Verification items for the finished model (mm, model axes). A direction names the side the tool comes from. Coordinates: 2 decimals unless noted, no trailing zeros. Write each loop counter-clockwise with the first axis right and the second up, starting at its lowest first coordinate (ties: lowest second). Pieces come first, ordered by that corner, then holes. Notation, with made-up numbers: M 27,33 L 65,33 A24 ccw 65,70 Z; hole C 14.5,77.25 d3. An arc over 180 degrees is marked long. One line per item, written item: value.
Autodesk Inventor part; units mm, degrees
ref_plane "YZ Plane" through (0, 0, 0) normal (1, 0, 0) x (0, 1, 0)
ref_plane "XZ Plane" through (0, 0, 0) normal (0, 1, 0) x (-1, 0, 0)
ref_plane "XY Plane" through (0, 0, 0) normal (0, 0, 1) x (1, 0, 0)
sketch "Sketch1" plane through (0, 0, 0) normal (0, 1, 0) x (-1, 0, 0)
  line L0 (0, 0) -> (-94, 0)
  line L1 (-94, 0) -> (-94, -87)
  line L2 (-94, -87) -> (0, -87)
  line L3 (0, -87) -> (0, 0)
  dimension "d0" = 94
  dimension "d1" = 87
extrude "Extrusion1" add sketch "Sketch1" along normal blind 2
sketch "Sketch2" plane through (0, 0, 0) normal (0, 0, 1) x (1, 0, 0)
  line L0 (94, 2) -> (0, 2)
  line L1 (-0.0001, 2) -> (94, 2)
  line L2 (94, 2) -> (99, 7)
  line L3 (94, 2) -> (101.071, 2) construction
  line L4 (94, 0) -> (99, 5)
  line L5 (99, 5) -> (114, 5)
  line L6 (114, 5) -> (114, 7)
  line L7 (114, 7) -> (99, 7)
  line L8 (94, 0) -> (94, 2)
  line L9 (94, 0) -> (94, 2)
  point P0 (0, 0)
  dimension "d4" = 7.071
  dimension "d5" = 45
  dimension "d6" = 7.071
  dimension "d7" = 15
  dimension "d8" = 2
extrude "Extrusion2" add sketch "Sketch2" against normal blind 87
sketch "Sketch3" plane through (99, 7, 0) normal (0, 1, 0) x (1, 0, 0)
  line L0 (15, 0) -> (0, 0)
  line L1 (15, 0) -> (20, 5)
  line L2 (15, 0) -> (22.071, 0) construction
  line L3 (20, 5) -> (20, 82)
  line L4 (0, 87) -> (15, 87)
  line L5 (20, 82) -> (15, 87)
  line L6 (15, 0) -> (15, 87)
  point P0 (-99, 0)
  dimension "d11" = 7.071
  dimension "d12" = 45
  dimension "d13" = 77
extrude "Extrusion3" add sketch "Sketch3" against normal blind 2
sketch "Sketch4" plane through (0, 2, 0) normal (0, 1, 0) x (1, 0, 0)
  line L0 (0, 0) -> (94, 0)
  line L1 (0, 0) -> (0, 4)
  line L2 (0, 87) -> (0, 0)
  line L3 (0, 4) -> (94, 4)
  line L4 (0, 4) -> (44, 4)
  line L5 (44, 4) -> (44, 14)
  line L6 (44, 14) -> (69, 14)
  line L7 (69, 14) -> (69, 4)
  dimension "d16" = 4
  dimension "d17" = 44
  dimension "d18" = 10
  dimension "d19" = 25
extrude "Extrusion4" cut sketch "Sketch4" against normal blind 10
ref_plane "Work Plane1" through (0, -2, 0) normal (0, -1, 0) x (1, 0, 0)
sketch "Sketch6" plane through (0, -2, 0) normal (0, -1, 0) x (1, 0, 0)
  line L0 (44, -4) -> (44, -14)
  line L1 (44, -4) -> (44, -2)
  line L2 (0, 0) -> (94, 0)
  line L3 (44, -2) -> (42, -2)
  line L4 (42, -2) -> (71, -2)
  line L5 (71, -2) -> (71, -16)
  line L6 (71, -16) -> (42, -16)
  line L7 (42, -16) -> (42, -2)
  line L8 (44, -4) -> (69, -4)
  line L9 (44, -14) -> (69, -14)
  line L10 (69, -14) -> (69, -4)
  line L11 (69, -4) -> (44, -4)
  line L12 (44, -4) -> (44, -14)
  dimension "d23" = 2
  dimension "d24" = 2
  dimension "d25" = 29
  dimension "d26" = 14
extrude "Extrusion5" add sketch "Sketch6" against normal blind 2
chamfer "Chamfer1" distance 2 angle 45 4 edges at (44, 2, -9) (56.5, 2, -14) (69, 2, -9) (56.5, 2, -4)
sketch "Sketch8" plane through (0, 2, 0) normal (0, 1, 0) x (1, 0, 0)
  line L0 (0, 0) -> (0, 25)
  line L1 (0, 87) -> (0, 0)
  line L2 (0, 25) -> (30, 25)
  circle A0 centre (30, 25) radius 7.5
  line L3 (30, 17.5) -> (30, 32.5)
  line L4 (37.5, 25) -> (22.5, 25)
  circle A1 centre (30, 25) radius 6
  line L5 (37.5, 25) -> (30, 25)
  line L6 (30, 25) -> (24, 25)
  line L7 (30, 25) -> (33.75, 25)
  line L8 (30, 25) -> (31.875, 25)
  line L9 (30, 25) -> (30.9375, 25)
  line L10 (30.9375, 25) -> (30.9375, 32.4412)
  line L11 (30.9375, 25) -> (28.9715, 25)
  line L12 (28.9715, 25) -> (28.9715, 32.4291)
  line L13 (30.9375, 25) -> (30.9375, 17.5588)
  line L14 (28.9715, 25) -> (28.9715, 17.5709)
  line L15 (30, 25) -> (30, 24.017)
  line L16 (30, 24.017) -> (30, 25.983)
  line L17 (37.4353, 25.983) -> (22.5647, 25.983)
  line L18 (37.4353, 24.017) -> (22.5647, 24.017)
  point P0 (30.9375, 24.017)
  point P1 (30.9375, 25.983)
  point P2 (28.9715, 25.983)
  point P3 (28.9715, 24.017)
  point P4 (24.0811, 25.983)
  point P5 (28.9715, 30.9112)
  point P6 (24.0811, 24.017)
  point P7 (28.9715, 19.0888)
  point P8 (35.9189, 24.017)
  point P9 (30.9375, 19.0737)
  point P10 (35.9189, 25.983)
  point P11 (30.9375, 30.9263)
  dimension "d34" = 15
  dimension "d35" = 12
  dimension "d32" = 25
  dimension "d33" = 30
  dimension "d36" = 1.966
  dimension "d37" = 0.983
  dimension "d38" = 1.966
extrude "Extrusion6" cut sketch "Sketch8" against normal blind 2 contours A0 L12 A1 L17 | L18 A1 L14 A0 | L12 L17 L3 L2 | L2 L3 L18 L14 | L4 L13 L18 L3 | L3 L17 L10 L4 | A0 L17 A1 L10 | L13 A1 L18 A0
sketch "Sketch9" plane through (0, 2, 0) normal (0, 1, 0) x (1, 0, 0)
  line L0 (0, 0) -> (0, 43)
  line L1 (0, 87) -> (0, 0)
  line L2 (0, 43) -> (21, 43)
  circle A0 centre (21, 43) radius 2.5
  line L3 (0, 0) -> (0, 52)
  line L4 (0, 52) -> (21, 52)
  circle A1 centre (21, 52) radius 2.5
  line L5 (0, 0) -> (0, 65)
  line L6 (0, 65) -> (21, 65)
  circle A2 centre (21, 65) radius 5
  dimension "d41" = 43
  dimension "d42" = 21
  dimension "d43" = 90
  dimension "d44" = 5
  dimension "d45" = 52
  dimension "d46" = 5
  dimension "d47" = 65
  dimension "d48" = 21
  dimension "d49" = 10
extrude "Extrusion7" cut sketch "Sketch9" against normal blind 2
sketch "Sketch10" plane through (0, 2, 0) normal (0, 1, 0) x (1, 0, 0)
  line L0 (0, 87) -> (0, 0)
  line L1 (0, 0) -> (43, 0)
  line L2 (0, 0) -> (94, 0)
  line L3 (43, 0) -> (43, 45)
  line L4 (71, 2) -> (42, 2)
  line L5 (71, 2) -> (70, 2)
  line L6 (70, 2) -> (70, 45)
  line L7 (70, 45) -> (74, 45) construction
  line L8 (70, 45) -> (70, 65)
  line L9 (70, 45) -> (90, 45) construction
  line L10 (70, 65) -> (67.7057, 68.2766)
  line L11 (67.7057, 68.2766) -> (45.2943, 68.2766)
  line L12 (43, 45) -> (43, 65)
  line L13 (43, 65) -> (45.2943, 68.2766)
  line L14 (70, 45) -> (70, 25)
  line L15 (70, 25) -> (66.8775, 22.5)
  line L16 (43, 45) -> (43, 25)
  line L17 (43, 25) -> (46.1225, 22.5)
  line L18 (46.1225, 22.5) -> (66.8775, 22.5)
  line L19 (66.8775, 22.5) -> (66.8775, 24.5)
  line L20 (70, 25) -> (68, 25)
  line L21 (68, 25) -> (66.8775, 24.5)
  line L22 (70, 65) -> (68, 65)
  line L23 (67.7057, 68.2766) -> (67.7057, 66.2766)
  line L24 (45.2943, 68.2766) -> (45.2943, 66.2766)
  line L25 (43, 65) -> (45, 65)
  line L26 (46.1225, 22.5) -> (46.1225, 24.5)
  line L27 (43, 25) -> (45, 25)
  line L28 (45, 25) -> (45, 65)
  line L29 (45, 65) -> (45.2943, 66.2766)
  line L30 (45.2943, 66.2766) -> (67.7057, 66.2766)
  line L31 (67.7057, 66.2766) -> (68, 65)
  line L32 (68, 65) -> (68, 25)
  line L33 (66.8775, 24.5) -> (46.1225, 24.5)
  line L34 (46.1225, 24.5) -> (45, 25)
  dimension "d52" = 43
  dimension "d53" = 45
  dimension "d54" = 1
  dimension "d58" = 20
  dimension "d59" = 90
  dimension "d60" = 20
  dimension "d61" = 4
  dimension "d62" = 20
  dimension "d63" = 4
  dimension "d64" = 2
  dimension "d65" = 2
  dimension "d66" = 2
  dimension "d67" = 2
  dimension "d68" = 2
  dimension "d69" = 2
  dimension "d70" = 2
  dimension "d71" = 2
extrude "Extrusion8" cut sketch "Sketch10" against normal blind 2 contours L28 L29 L30 L31 L32 L21 L33 L34
chamfer "Chamfer2" distance 2 angle 45 8 edges at (45, 2, -45) (45.5612, 2, -24.75) (56.5, 2, -24.5) (67.4388, 2, -24.75) (68, 2, -45) (56.5, 2, -66.2766) (45.1472, 2, -65.6383) (67.8528, 2, -65.6383)
sketch "Sketch11" plane through (0, 2, 0) normal (0, 1, 0) x (1, 0, 0)
  line L0 (45.6972, 22.5) -> (67.3028, 22.5)
  line L1 (67.3028, 22.5) -> (45.6972, 22.5)
  line L2 (43, 23.7014) -> (45.6972, 22.5)
  line L3 (45.6972, 22.5) -> (43, 23.7014)
  line L4 (43, 23.7014) -> (45, 25)
  line L5 (43, 65.2276) -> (43, 23.7014)
  line L6 (43, 23.7014) -> (43, 65.2276)
  line L7 (43.7029, 68.2766) -> (45.2943, 66.2766)
  line L8 (43, 65.2276) -> (43.7029, 68.2766)
  line L9 (70, 23.7014) -> (70, 65.2276)
  line L10 (43, 23.7014) -> (70, 23.7014)
  line L11 (70, 65.2276) -> (68, 65)
  line L12 (43, 65.2276) -> (70, 65.2276)
  line L13 (69.2971, 68.2766) -> (43.7029, 68.2766)
  line L14 (43.7029, 68.2766) -> (69.2971, 68.2766)
  line L15 (45.6972, 22.5) -> (67.3028, 22.5)
  line L16 (43, 65.2276) -> (43.7029, 68.2766)
  line L17 (43.7029, 68.2766) -> (69.2971, 68.2766)
  line L18 (46.1225, 24.5) -> (66.8775, 24.5)
  line L19 (66.8775, 24.5) -> (46.1225, 24.5)
  line L20 (45.6972, 22.5) -> (43, 23.7014)
  line L21 (43, 23.7014) -> (43, 65.2276)
  line L22 (43, 65.2276) -> (43.7029, 68.2766)
  line L23 (69.2971, 68.2766) -> (43.7029, 68.2766)
  line L24 (70, 65.2276) -> (69.2971, 68.2766)
  line L25 (69.2971, 68.2766) -> (70, 65.2276)
  line L26 (67.3028, 22.5) -> (70, 23.7014)
  line L27 (67.3028, 22.5) -> (70, 23.7014)
  line L28 (68, 25) -> (68, 65)
  line L29 (66.8775, 24.5) -> (68, 25)
  line L30 (68, 65) -> (68, 25)
  line L31 (66.8775, 24.5) -> (46.1225, 24.5)
  line L32 (45, 25) -> (46.1225, 24.5)
  line L33 (46.1225, 24.5) -> (45, 25)
  line L34 (45, 25) -> (45, 65)
  line L35 (45, 65) -> (45.2943, 66.2766)
  line L36 (67.7057, 66.2766) -> (45.2943, 66.2766)
  line L37 (68, 65) -> (67.7057, 66.2766)
  point P0 (0, 0)
sketch "Sketch12" plane through (99, 7, 0) normal (0, 1, 0) x (1, 0, 0)
  line L0 (20, 5) -> (15, 0)
  line L1 (20, 5) -> (0, 5)
  line L2 (0, 0) -> (0, 87)
  line L3 (15, 87) -> (20, 82)
  line L4 (20, 82) -> (0, 82)
  line L5 (10, 82) -> (10, 5)
  line L6 (0, 5) -> (10, 5)
  line L7 (5, 5) -> (5, 82)
  line L8 (10, 5) -> (20, 5)
  line L9 (15, 5) -> (15, 82)
  line L10 (10, 5) -> (15, 5)
  line L11 (10, 5) -> (5, 5)
  line L12 (7.5, 5) -> (7.5, 82)
  line L13 (12.5, 82) -> (12.5, 5)
  point P0 (-99, 0)
  point P1 (7.5, 5)
  point P2 (5, 5)
  point P3 (12.5, 5)
  point P4 (15, 5)
extrude "Extrusion9" cut sketch "Sketch12" against normal blind 2 contours L1 L13 L4 L9 | L1 L7 L4 L12
sketch "Sketch13" plane through (0, 0, 0) normal (0, -1, 0) x (1, 0, 0)
  circle A0 centre (21, -52) radius 2.5
  circle A1 centre (21, -52) radius 3.5
  circle A2 centre (21, -43) radius 2.5
  circle A3 centre (21, -43) radius 3.5
  circle A4 centre (21, -65) radius 5
  circle A5 centre (21, -65) radius 7.5
  point P0 (0, 0)
  dimension "d79" = 7
  dimension "d80" = 7
  dimension "d81" = 15
extrude "Extrusion10" cut sketch "Sketch13" against normal blind 1
sketch "Sketch14" plane through (0, 0, 0) normal (0, -1, 0) x (1, 0, 0)
  circle A0 centre (21, -65) radius 5
  circle A1 centre (21, -65) radius 5
  point P0 (0, 0)
equation "\"BendRadius\" = Thickness"
equation "\"BendReliefWidth\" = Thickness"
equation "\"BendReliefDepth\" = 0.5 * Thickness"
equation "\"CornerReliefSize\" = 4 * Thickness"
equation "\"MinimumRemnant\" = 2 * Thickness"
equation "\"TransitionRadius\" = BendRadius"
equation "\"JacobiRadiusSize\" = BendRadius"
equation "\"GapSize\" = Thickness"
properties part number "Part2edd"
Item 1: Cross-section at A-A, the plane z = -12. Enter the section's corners in (x, y), and give its area (3 significant figures).
The answers:
outline: M 0,0 L 42,0 L 42,-2 L 44,-2 L 44,0 L 42,2 L 0,2 Z; M 69,-2 L 71,-2 L 71,0 L 94,0 L 99,5 L 104,5 L 104,7 L 99,7 L 94,2 L 71,2 L 69,0 Z; M 106.5,5 L 111.5,5 L 111.5,7 L 106.5,7 Z; M 114,5 L 119,5 L 119,7 L 114,7 Z
area: 182 mm²
Item 2: Go/stop test with flat-tipped pins: P1, Ø0.6, axis at y = 6, z = -40.5, coming from the -X side; P2, Ø12, axis at x = 38, z = -66.5, coming from the -Y side; P3, Ø1.6, axis at y = -1.5, z = -7, coming from the -X side; P4, Ø2, axis at x = 59.5, y = -0.5, coming from the +Z side. Record where each tip stops, or that it passes through.
The answers:
P1: stops at x = 97.7
P2: stops at y = 0
P3: stops at x = 42
P4: stops at z = 0
Item 3: Cross-section at B-B, the plane x = 21. Enter the section's corners in (y, z), and give its area (3 significant figures).
The answers:
outline: M 0,-87 L 2,-87 L 2,-70 L 1,-70 L 1,-72.5 L 0,-72.5 Z; M 0,-57.5 L 1,-57.5 L 1,-60 L 2,-60 L 2,-54.5 L 1,-54.5 L 1,-55.5 L 0,-55.5 Z; M 0,-48.5 L 1,-48.5 L 1,-49.5 L 2,-49.5 L 2,-45.5 L 1,-45.5 L 1,-46.5 L 0,-46.5 Z; M 0,-39.5 L 1,-39.5 L 1,-40.5 L 2,-40.5 L 2,0 L 0,0 Z
area: 125 mm²
Item 4: Draft check along X on faces 1 (the face through (116, 6, -2)), 2 (the face through (34.263, 1.014, -29.222)), 3 (the face through (109, 5, -44)). Enter one of: released by +X, released by -X, zero draft, split by the parting line, or undercut.
The answers:
face 1: released by +X
face 2: undercut
face 3: zero draft
Item 5: Access from +Z, -Z, +X, -X, +Y, -Y to the whole of each face (thin tool, end or side, straight path). Record for faces 4 (the face through (37, 2, -43)), 5 (the face through (25.705, 1.014, -20.811)), 6 (the face through (15.5, 0.5, -59.9)), 7 (the face through (44.95, 1.21, -23.7)).
The answers:
face 4: +Z, -Z, -X, +Y
face 5: +Y, -Y
face 6: -Y
face 7: +Y
Item 6: Cross-section at C-C, the plane z = -43. Give the number of separate pieces and of enclosed holes in the cut face, and give its area (3 significant figures).
The answers:
separate pieces: 5
enclosed holes: 0
area: 166 mm²
Item 7: Cross-section at D-D, the plane y = 3.5. Enter the section's corners in (x, z).
The answers:
outline: M 95.5,-87 L 97.5,-87 L 97.5,0 L 95.5,0 Z
Item 8: Scan lines: line 1 (Z direction, x = 21, y = 0.6); line 2 (Z direction, x = 21, y = 1.6); line 3 (X direction, y = -1.5, z = -11). Record each from-to range of solid material in increasing order.
The answers:
line 1: z = -87 to -72.5, -57.5 to -55.5, -48.5 to -46.5, -39.5 to 0
line 2: z = -87 to -70, -60 to -54.5, -49.5 to -45.5, -40.5 to 0
line 3: x = 42 to 44, 69 to 71
